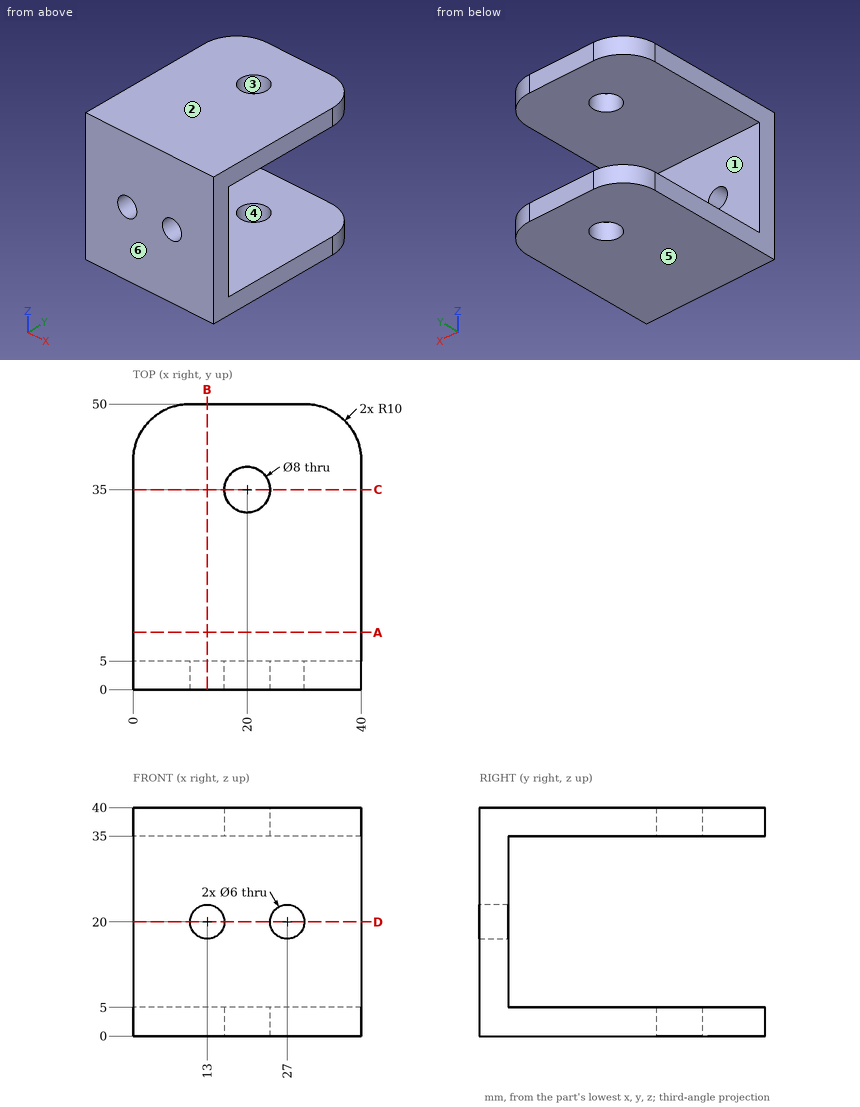
Source: three-view drawing plus pictorial views. Frame: mm from the lowest corner of the part. A direction names the side the tool comes from. Give positions to 0.01 mm unless a question says otherwise; leave off trailing zeros. Write each loop counter-clockwise with the first axis right and the second up, starting at its lowest first coordinate (ties: lowest second). Pieces come first, ordered by that corner, then holes. Notation, with made-up numbers: (36, 33.5) -> (88, 33.5) arc R19 ccw to (88, 38.5) -> close; hole circle Ø8 at (66.25, -38). An arc over 180 degrees is marked (long way). Write item = value, one per line.
Q1. Cut plane D-D on z = 20. Return loops of the section in (x, y), then the cut area to 3 significant figures.
Here are the results:
outline = (0, 0) -> (10, 0) -> (10, 5) -> (0, 5) -> close; (16, 0) -> (24, 0) -> (24, 5) -> (16, 5) -> close; (30, 0) -> (40, 0) -> (40, 5) -> (30, 5) -> close
area = 140 mm²
Q2. Reachability of the marked faces 1 and 2 from +Z, -Z, +X, -X, +Y, -Y: full face, straight path, thin tool, end or side. Return the list, or none.
Here are the results:
face_1 = +X, -X, +Y
face_2 = +Z, +X, -X, +Y, -Y
Q3. Line query: line 1 (X direction, y = 2, z = 20); line 2 (Z direction, x = 10.5, y = 10.5); line 3 (Y direction, x = 20, z = 1). Output: solid intervals per line, ascending. Write a range as from..to.
Here are the results:
line_1 = 0..10, 16..24, 30..40
line_2 = 0..5, 35..40
line_3 = 0..31, 39..50
Q4. First-contact query: pin 1 (24 mm diameter, centred on x = 26, z = 14.5, fed in from +Y); pin 2 (8 mm diameter, centred on x = 13, z = 20, fed in from +Y); pin 3 (6.5 mm diameter, centred on x = 20, y = 35, fed in from +Z). Flat tips, straight axial feed; report the tip coordinate or a pass-through.
Here are the results:
pin_1 = 50
pin_2 = 5
pin_3 = through
Q5. Mould query, pull axis Y, two halves, no side actions, for the marked faces 3, 4, 5 and 6. Classes: +Y half, -Y half, draft (parallel to the pull), parting line (faces both ways), or undercut.
Here are the results:
face_3 = undercut
face_4 = undercut
face_5 = draft
face_6 = -Y half
Q6. Cut plane A-A on y = 10. Return loops of the section in (x, z), then the cut area to 3 significant figures.
Here are the results:
outline = (0, 0) -> (40, 0) -> (40, 5) -> (0, 5) -> close; (0, 35) -> (40, 35) -> (40, 40) -> (0, 40) -> close
area = 400 mm²
Q7. Cut plane C-C on y = 35. Return loops of the section in (x, z), then the cut area to 3 significant figures.
Here are the results:
outline = (0, 0) -> (16, 0) -> (16, 5) -> (0, 5) -> close; (0, 35) -> (16, 35) -> (16, 40) -> (0, 40) -> close; (24, 0) -> (40, 0) -> (40, 5) -> (24, 5) -> close; (24, 35) -> (40, 35) -> (40, 40) -> (24, 40) -> close
area = 320 mm²
Q8. Cut plane B-B on x = 13. Return loops of the section in (y, z), then the cut area to 3 significant figures.
Here are the results:
outline = (0, 0) -> (50, 0) -> (50, 5) -> (5, 5) -> (5, 17) -> (0, 17) -> close; (0, 23) -> (5, 23) -> (5, 35) -> (50, 35) -> (50, 40) -> (0, 40) -> close
area = 620 mm²
